Check sheet for the modelled part. Datum: model origin and axes. Units: mm. A direction names the side the tool comes from. Coordinates: 2 decimals unless noted, no trailing zeros. Loops run counter-clockwise (first coordinate to the right, second up) from the corner with the lowest first, then second, coordinate; pieces in that order, holes last. Notation, with made-up numbers: M 42,53.5 L 90,53.5 A21 ccw 90,64.5 Z; hole C -16.5,9.25 d2. An arc over 180 degrees is marked long. Use CSV: the item, a comma, the result in double quotes. Start each with the question number.
(1) Set-up check for faces 1 (the cylindrical face through (85.88, 95.78, 0.7)), 2 (the flat face through (155.696, 114.072, 0.7)): record each of +Z, -Z, +X, -X, +Y, -Y from which the full face is reachable in a straight line by a thin tool's end or side.
(2) Section check A-A on z = -31. Record the cut outline in (x, y).
(3) Scan lines: line 1 (Y direction, x = 67.5, z = 11); line 2 (Y direction, x = 116, z = -33.5); line 3 (Y direction, x = 78.5, z = -16.5). Record each from-to range of solid material in increasing order.
(4) Section check D-D on x = 65. Record the cut outline in (y, z).
(5) Go/stop test with flat-tipped pins: pin 1 Ø2 at (y, z) = (131.5, 5.5) entering from -X; pin 2 Ø5 at (y, z) = (117.5, 26.5) entering from +X; pin 3 Ø1 at (y, z) = (128.5, 0) entering from -X. Record where each tip stops, or that it passes through.
(6) Section check B-B on x = 84.5. Record the cut outline in (y, z), and give its area (3 significant figures).
(7) Section check C-C on y = 94. Record the cut outline in (x, z), and give its area (3 significant figures).
from build123d import *

# Parameters (mm, degrees)
EXTRUDE_1_DEPTH                = 50
SPLIT_BODIES_1_SURFACE_1_BACK  = 235.567
SPLIT_BODIES_1_SURFACE_1_DEPTH = 471.134
SPLIT_BODIES_1_SURFACE_2_BACK  = 235.567
SPLIT_BODIES_1_SURFACE_2_DEPTH = 471.134


with BuildPart() as part:
    # 草图1 → 凸台-拉伸1 (new, symmetric)
    with BuildSketch(Plane.XY):
        with BuildLine():
            Line((56.67204093, 43.504108875), (36.476006197, 29.147891414))
            Line((36.476006197, 29.147891414), (0, 29.147891414))
            Line((0, 29.147891414), (0, 0))
            Line((0, 0), (144.001, 0))
            Line((144.001, 0), (134.529857437, 27.122156161))
            Line((134.529857437, 27.122156161), (117.072161438, 27.122156161))
            Line((117.072161438, 27.122156161), (123.353516134, 49.257428232))
            Line((123.353516134, 49.257428232), (139.303205185, 49.257428232))
            Line((139.303205185, 49.257428232), (150.141177621, 92.108587215))
            ThreePointArc((150.141177621, 92.108587215), (153.228333696, 99.503580273), (154.028196985, 107.477078481))
            Line((154.028196985, 107.477078481), (157.411382406, 120.853511867))
            ThreePointArc((157.411382406, 120.853511867), (156.730372482, 125.265422842), (153.08647989, 127.844333418))
            Line((153.08647989, 127.844333418), (137.369721749, 131.276874543))
            ThreePointArc((137.369721749, 131.276874543), (132.648572458, 132.768940094), (127.735239934, 133.381046075))
            Line((127.735239934, 133.381046075), (89.661, 141.696462857))
            ThreePointArc((89.661, 141.696462857), (71.40391268, 133.595205289), (73.639067543, 113.746888123))
            ThreePointArc((73.639067543, 113.746888123), (86.014043833, 95.502710926), (92.496172884, 74.432066828))
            Line((92.496172884, 74.432066828), (56.67204093, 74.432066828))
            Line((56.67204093, 74.432066828), (56.67204093, 43.504108875))
        make_face()
    extrude(amount=EXTRUDE_1_DEPTH, both=True)


with BuildPart() as body_2:
    # Split Bodies 1: the piece behind the surface
    add(part.part)
    # Split Bodies 1 surface: a surface, the sketch's curves swept straight by 471.134 mm
    with BuildLine(Plane.XY.offset(50).offset(-SPLIT_BODIES_1_SURFACE_1_BACK), mode=Mode.PRIVATE) as split_bodies_1_surface_1_path:
        Line((123.353516134, 49.257428232), (56.67204093, 49.257428232))
    split_bodies_1_surface_1 = Shell.extrude(split_bodies_1_surface_1_path.wire(), (0 * SPLIT_BODIES_1_SURFACE_1_DEPTH, 0 * SPLIT_BODIES_1_SURFACE_1_DEPTH, 1 * SPLIT_BODIES_1_SURFACE_1_DEPTH))
    split(bisect_by=split_bodies_1_surface_1, keep=Keep.BOTTOM)


with BuildPart() as part_1:
    add(part.part)

    # Split Bodies 1: split by a surface, the side it looks to stays
    # Split Bodies 1 surface: a surface, the sketch's curves swept straight by 471.134 mm
    with BuildLine(Plane.XY.offset(50).offset(-SPLIT_BODIES_1_SURFACE_2_BACK), mode=Mode.PRIVATE) as split_bodies_1_surface_2_path:
        Line((123.353516134, 49.257428232), (56.67204093, 49.257428232))
    split_bodies_1_surface_2 = Shell.extrude(split_bodies_1_surface_2_path.wire(), (0 * SPLIT_BODIES_1_SURFACE_2_DEPTH, 0 * SPLIT_BODIES_1_SURFACE_2_DEPTH, 1 * SPLIT_BODIES_1_SURFACE_2_DEPTH))
    split(bisect_by=split_bodies_1_surface_2, keep=Keep.TOP)


solid = body_2.part
Outcome:
1,face 1,"+Z, -Z, -X"
1,face 2,"+Z, -Z, +X, -Y"
2,outline,"M 56.67,49.26 L 139.3,49.26 L 150.14,92.11 A27.22 ccw 154.03,107.48 L 157.41,120.85 A5.72 ccw 153.09,127.84 L 137.37,131.28 A27.22 ccw 127.74,133.38 L 89.66,141.7 A16.89 ccw 73.64,113.75 A74.36 cw 92.5,74.43 L 56.67,74.43 Z"
3,line 1,"y = 49.26 to 74.43"
3,line 2,"y = 49.26 to 135.94"
3,line 3,"y = 49.26 to 74.43, 107.9 to 140.3"
4,outline,"M 49.26,-50 L 74.43,-50 L 74.43,50 L 49.26,50 Z"
5,pin 1,"stops at x = 70.02"
5,pin 2,"stops at x = 157.2"
5,pin 3,"stops at x = 69.4"
6,outline,"M 49.26,-50 L 74.43,-50 L 74.43,50 L 49.26,50 Z; M 98.49,-50 L 142.01,-50 L 142.01,50 L 98.49,50 Z"
6,area,"6,870 mm²"
7,outline,"M 86.71,-50 L 151.18,-50 L 151.18,50 L 86.71,50 Z"
7,area,"6,450 mm²"
